from build123d import *

# Parameters (mm, degrees)
SKETCH_1_R      = 2.5
EXTRUDE_1_DEPTH = 9
SKETCH_4_W      = 1.07639592
SKETCH_4_H      = 0.25
SKETCH_5_R      = 2.5
EXTRUDE_3_DEPTH = 0.24
SKETCH_6_R      = 0.5


with BuildPart() as part:
    # 草图1 → 凸台-拉伸1 (new body)
    with BuildSketch(Plane(origin=(0, 0, 0), x_dir=(1, 0, 0), z_dir=(0, 1, 0))):
        with Locations(Location((0, 0, 0), (0, 0, 270))):
            Circle(SKETCH_1_R)
    extrude(amount=EXTRUDE_1_DEPTH)

    # 草图4 → 切除-旋转1 (revolve, cut)
    with BuildSketch(Plane.XY, mode=Mode.PRIVATE) as cut_revolve_1_sk:
        with Locations((-2.83819796, 6.898899293)):
            Rectangle(SKETCH_4_W, SKETCH_4_H)
    revolve(cut_revolve_1_sk.sketch.rotate(Axis((0, 9.45, 0), (0, -1, 0)), 270), axis=Axis((0, 9.45, 0), (0, -1, 0)), mode=Mode.SUBTRACT)

    # 草图5 → 凸台-拉伸3 (add)
    with BuildSketch(Plane(origin=(0, 6.773899293, 0), x_dir=(1, 0, 0), z_dir=(0, 1, 0))):
        with Locations(Location((0, 0, 0), (0, 0, 270))):
            Circle(SKETCH_5_R)
    extrude(amount=EXTRUDE_3_DEPTH)

    # 扫描1: sweep along a path in 草图7
    with BuildLine(Plane(origin=(0, 0, 0), x_dir=(0, 0, -1), z_dir=(1, 0, 0))) as sweep_1_path:
        Line((-4.5, -2.75), (-1.5, -2.75))
        ThreePointArc((-1.5, -2.75), (-0.085786438, -2.164213562), (0.5, -0.75))
        Line((0.5, -0.75), (0.5, 0))
    # 草图6 → 扫描1 (sweep)
    with BuildSketch(Plane.XZ):
        Circle(SKETCH_6_R)
    sweep_1 = sweep(path=sweep_1_path.line)

    # 镜向1: 扫描1 across plane
    add(sweep_1.mirror(Plane.ZX.offset(4.5)))


solid = part.part
Work out the finished part from the listing and answer in its coordinate system (mm). A direction names the side the tool comes from. Coordinates: 2 decimals unless noted, no trailing zeros. Loops run counter-clockwise (first coordinate to the right, second up) from the corner with the lowest first, then second, coordinate; pieces in that order, holes last. Notation, with made-up numbers: (42.5, 38) -> (75.5, 38) arc R23 cw to (75.5, 59) -> close; hole circle Ø9 at (-35, -39.5). An arc over 180 degrees is marked (long way). Answer as CSV lines item,"result".
1) The part is cut by section C-C (z = 3.5). Give the vertices of the cut face in (x, y).
A:
outline,"circle Ø1 at (0, -2.25); circle Ø1 at (0, 11.25)"
2) For faces 1 (the face through (-0.065, -2.746, 2.979)), 2 (the face through (-0.108, -0.37, 0.488)), 3 (the face through (0, 11, 4.5)), determine the directions among +Z, -Z, +X, -X, +Y, -Y from which every point of the face is accessible in a straight line to the end or side of a thin tool.
A:
face 1,"+Z"
face 2,"none"
face 3,"+Z, +X, -X, +Y, -Y"
3) The part is cut by section A-A (z = 1.75). State how many separate pieces and enclosed holes the cut face has, and give its area (3 significant figures).
A:
separate pieces,"3"
enclosed holes,"0"
area,"33.7 mm²"
4) For a pull along Y with two mould halves and no side action, classify faces 4 (the face through (0, -2, 4.5)), 5 (the face through (0.231, 10.806, 2.979)) as released by +Y, released by -Y, zero draft, split by the parting line, or undercut.
A:
face 4,"zero draft"
face 5,"undercut"
5) Flat-ended cylindrical pins translate along their axes: pin 1 (1 mm diameter, centred on y = 8, z = -1.5, fed in from +X); pin 2 (4 mm diameter, centred on y = 9, z = 3.5, fed in from -X); pin 3 (1 mm diameter, centred on y = 1, z = -1.5, fed in from -X). Find the tip coordinate at first contact, or state that the pin passes through.
A:
pin 1,"stops at x = 2.29"
pin 2,"stops at x = -2"
pin 3,"stops at x = -2.29"
6) Straight lines are drawn through the part: probe 1 along Y at (x, z) = (0.15, -1.75); probe 2 along Y at (x, z) = (-0.25, 3.75); probe 3 along Z at (x, y) = (0.5, 5). For each, find the intervals that lie inside material, in ascending order.
A:
probe 1,"y = 0 to 9"
probe 2,"y = -2.68 to -1.82, 10.82 to 11.68"
probe 3,"z = -2.45 to 2.45"
7) The part is cut by section D-D (y = 8). Give the vertices of the cut face in (x, z), and give its area (3 significant figures).
A:
outline,"circle Ø5 at (0, 0)"
area,"19.6 mm²"
